Geometry check sheet. Reference: the model listing, model coordinates, mm. Give positions to 0.01 mm unless a question says otherwise; leave off trailing zeros. Order: outer loops, then holes, each group sorted by start corner. A loop starts at its lowest first (then second) coordinate and runs counter-clockwise, first axis right, second up. Notation, with made-up numbers: M 65.25,81.5 L 111.25,81.5 A17 ccw 111.25,87.5 Z; hole C 83,13.5 d6. An arc over 180 degrees is marked long. Answer as a JSON object with one key per item and string values. Group by question number.
Autodesk Inventor part; units mm, degrees
ref_plane "YZ Plane" through (0, 0, 0) normal (1, 0, 0) x (0, 1, 0)
ref_plane "XZ Plane" through (0, 0, 0) normal (0, 1, 0) x (-1, 0, 0)
ref_plane "XY Plane" through (0, 0, 0) normal (0, 0, 1) x (1, 0, 0)
sketch "Sketch1" plane through (0, 0, 0) normal (0, 0, 1) x (1, 0, 0)
  line L0 (-50.8, -28.575) -> (50.8, -28.575)
  line L1 (50.8, -28.575) -> (50.8, 28.575)
  line L2 (50.8, 28.575) -> (-50.8, 28.575)
  line L3 (-50.8, 28.575) -> (-50.8, -28.575)
  line L4 (-50.8, -28.575) -> (50.8, 28.575) construction
  line L5 (50.8, -28.575) -> (-50.8, 28.575) construction
  circle A0 centre (-46.99, 24.765) radius 1.5
  line L6 (-50.8, 0) -> (50.8, 0) construction
  line L7 (0, 28.575) -> (0, -28.575) construction
  circle A1 centre (-46.99, -24.765) radius 1.5
  circle A2 centre (46.99, 24.765) radius 1.5
  circle A3 centre (46.99, -24.765) radius 1.5
  point P0 (0, 0)
  dimension "d2" = 101.6
  dimension "d4" = 57.15
  dimension "d5" = 49.53
  dimension "d6" = 3
  dimension "d7" = 93.98
extrude "Extrusion1" add sketch "Sketch1" along normal blind 1
properties part number "Microzed01" material "PCB(1)"
1. Depth check by flat-ended pin: pin 1 (1.8 mm diameter, centred on x = 46.99, y = -24.765, fed in from -Z). Enter the tip coordinate at first touch or a pass-through.
2. Release check for a two-part mould opening along X. For faces 1 (the flat face through (-1, 0, 0)), 2 (the cylindrical face through (48.42, -25.22, 0.49)) record: released by +X, released by -X, zero draft, split by the parting line, or undercut.
3. Thickness scan on line 1 along Y through (x, z) = (-46.99, 0.7) (3 decimals); line 2 along X through (y, z) = (-25, 0.2); line 3 along X through (y, z) = (24, 0.55). Record the ranges inside material, lowest first. Write a range as [from, to].
4. Cross-section at A-A (x = 46.99). Record the cut outline in (y, z) (3 decimals).
Report:
{
 "1": {"pin 1": "passes through"},
 "2": {"face 1": "zero draft", "face 2": "undercut"},
 "3": {"line 1": "y = [-28.575, -26.265], [-23.265, 23.265], [26.265, 28.575]", "line 2": "x = [-50.8, -48.47], [-45.51, 45.51], [48.47, 50.8]", "line 3": "x = [-50.8, -48.28], [-45.7, 45.7], [48.28, 50.8]"},
 "4": {"outline": "M -28.575,0 L -26.265,0 L -26.265,1 L -28.575,1 Z; M -23.265,0 L 23.265,0 L 23.265,1 L -23.265,1 Z; M 26.265,0 L 28.575,0 L 28.575,1 L 26.265,1 Z"}
}
